Part model, mm, in its own coordinate system. Coordinates: 2 decimals unless noted, no trailing zeros. Write each loop counter-clockwise with the first axis right and the second up, starting at its lowest first coordinate (ties: lowest second). Pieces come first, ordered by that corner, then holes. Notation, with made-up numbers: (-15.75, 47) - (17.25, 47) arc R17 ccw to (17.25, 68) - close; hole circle Ø6 at (89, 29.5). An arc over 180 degrees is marked (long way). Use a Markdown table: item, result.
```python
from build123d import *

# Parameters (mm, degrees)
SKIZZE1_R                       = 4.75
LINEAR_AUSTRAGEN1_DEPTH         = 5
SKIZZE10_R                      = 57.5
SCHNITT_LINEAR_AUSTRAGEN3_DEPTH = 471.252591699
SKIZZE15_R                      = 4.25
SCHNITT_LINEAR_AUSTRAGEN5_DEPTH = 471.252591699
M6_GEWINDEBOHRUNG1_D            = 5
SKIZZE17_R                      = 4.5
SCHNITT_LINEAR_AUSTRAGEN7_DEPTH = 471.252591699


with BuildPart() as part:
    # Skizze1 → Linear austragen1 (new body)
    with BuildSketch(Plane.XY):
        with BuildLine():
            Line((100, 317.106054814), (100, -317.106054814))
            ThreePointArc((100, -317.106054814), (-332.5, 0), (100, 317.106054814))
        make_face()
        with Locations((56.088361386, 318.092904223)):
            Circle(SKIZZE1_R, mode=Mode.SUBTRACT)
        with Locations((56.088361386, -318.092904223)):
            Circle(SKIZZE1_R, mode=Mode.SUBTRACT)
        with Locations((-161.5, -279.726205422)):
            Circle(SKIZZE1_R, mode=Mode.SUBTRACT)
        with Locations((-303.520716514, -110.472506294)):
            Circle(SKIZZE1_R, mode=Mode.SUBTRACT)
        with Locations((-303.520716514, 110.472506294)):
            Circle(SKIZZE1_R, mode=Mode.SUBTRACT)
        with Locations((-161.5, 279.726205422)):
            Circle(SKIZZE1_R, mode=Mode.SUBTRACT)
    extrude(amount=LINEAR_AUSTRAGEN1_DEPTH)

    # Skizze10 → Schnitt-Linear austragen3 (cut, through all)
    with BuildSketch(Plane.XY.offset(5)):
        Circle(SKIZZE10_R)
    extrude(amount=-SCHNITT_LINEAR_AUSTRAGEN3_DEPTH, mode=Mode.SUBTRACT)

    # Skizze15 → Schnitt-Linear austragen5 (cut, through all)
    with BuildSketch(Plane.XY.offset(5)):
        with Locations((-45.961940777, 45.961940777)):
            Circle(SKIZZE15_R)
        with Locations((45.961940777, 45.961940777)):
            Circle(SKIZZE15_R)
        with Locations((45.961940777, -45.961940777)):
            Circle(SKIZZE15_R)
        with Locations((-45.961940777, -45.961940777)):
            Circle(SKIZZE15_R)
    extrude(amount=-SCHNITT_LINEAR_AUSTRAGEN5_DEPTH, mode=Mode.SUBTRACT)

    # M6 Gewindebohrung1 (through all)
    with Locations(Plane.XY.offset(5)):
        with Locations((78, -262), (78, -178), (78, 178), (78, 262)):
            Hole(M6_GEWINDEBOHRUNG1_D / 2)

    # Skizze17 → Schnitt-Linear austragen7 (cut, through all)
    with BuildSketch(Plane.XY.offset(5)):
        with Locations((87.5, -150)):
            Circle(SKIZZE17_R)
        with Locations((87.5, 150)):
            Circle(SKIZZE17_R)
    extrude(amount=-SCHNITT_LINEAR_AUSTRAGEN7_DEPTH, mode=Mode.SUBTRACT)


solid = part.part
```
Item 1: Band-saw the part on C-C, the plane z = 3.3. Count the separate pieces of the cut face and the enclosed holes in it, then the cut area to 3 significant figures.
From the geometry:
| item | result |
|---|---|
| separate pieces | 1 |
| enclosed holes | 17 |
| area | 228,000 mm^2 |
Item 2: Band-saw the part on A-A, the plane x = 0. Give the cut face in (y, z), then the cut area to 3 significant figures.
From the geometry:
| item | result |
|---|---|
| outline | (-332.5, 0) - (-57.5, 0) - (-57.5, 5) - (-332.5, 5) - close; (57.5, 0) - (332.5, 0) - (332.5, 5) - (57.5, 5) - close |
| area | 2,750 mm^2 |
Item 3: Band-saw the part on D-D, the plane x = -112. Give the cut face in (y, z).
From the geometry:
| item | result |
|---|---|
| outline | (-313.07, 0) - (313.07, 0) - (313.07, 5) - (-313.07, 5) - close |
Item 4: Two-plate mould, pull along X, no slides. Class faces 1 (the face through (-12.465, -56.133, 2.535)), 2 (the face through (-65, 5, 0)): pulls with the +X half, pulls with the -X half, needs draft (parallel to the pull), parting line crosses it, or undercut.
From the geometry:
| item | result |
|---|---|
| face 1 | undercut |
| face 2 | needs draft |
Item 5: Band-saw the part on B-B, the plane y = 0. Give the cut face in (x, z), then the cut area to 3 significant figures.
From the geometry:
| item | result |
|---|---|
| outline | (-332.5, 0) - (-57.5, 0) - (-57.5, 5) - (-332.5, 5) - close; (57.5, 0) - (100, 0) - (100, 5) - (57.5, 5) - close |
| area | 1,590 mm^2 |
Item 6: Drop flat-ended pins along their axis: P1, Ø4.5, axis at x = 78, y = 178, coming from the -Z side; P2, Ø13.5, axis at x = 45.96, y = -45.96, coming from the +Z side. Give the stop position or say it passes through.
From the geometry:
| item | result |
|---|---|
| P1 | through |
| P2 | z = 5 |
Item 7: Drill centre lines: probe 1 along Y at (x, z) = (-45, 1.7); probe 2 along Y at (x, z) = (-161.5, 3.1); probe 3 along X at (y, z) = (-1, 4.75). Where is each one in solid material? Low to high.
From the geometry:
| item | result |
|---|---|
| probe 1 | -329.44 to -50.1, -41.82 to -35.79, 35.79 to 41.82, 50.1 to 329.44 |
| probe 2 | -290.64 to -284.48, -274.98 to 274.98, 284.48 to 290.64 |
| probe 3 | -332.5 to -57.49, 57.49 to 100 |
